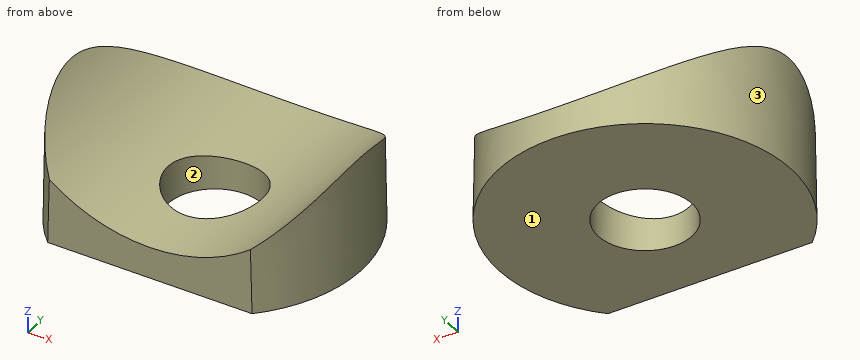
```python
from build123d import *

# Parameters (mm, degrees)
F0_R     = 14
F1_DEPTH = 12
F1_TAPER = 1
F2_R     = 16
F3_DEPTH = 16
F4_R     = 4.5
F5_DEPTH = 5
F7_DEPTH = 10.9201391502


with BuildPart() as f1:
    # F0 (on Top) → F1 (new body)
    with BuildSketch(Plane.XY):
        Circle(F0_R)
    extrude(amount=F1_DEPTH, taper=F1_TAPER)

    # F2 (on Front) → F3 (cut, symmetric)
    with BuildSketch(Plane.XZ):
        with Locations((0, 19)):
            Circle(F2_R)
    extrude(amount=F3_DEPTH, both=True, mode=Mode.SUBTRACT)

    # F4 (on face) → F5 (cut)
    with BuildSketch(Plane(origin=(0, 0, 0), x_dir=(1, 0, 0), z_dir=(0, 0, -1))):
        Circle(F4_R)
    extrude(amount=-F5_DEPTH, mode=Mode.SUBTRACT)

    # F6 (on face) → F7 (cut, through all)
    with BuildSketch(Plane(origin=(0, 0, 0), x_dir=(1, 0, 0), z_dir=(0, 0, -1))):
        with BuildLine():
            ThreePointArc((9.7979589711, 10), (0, 14), (-9.7979589711, 10))
            Line((-9.7979589711, 10), (9.7979589711, 10))
        make_face()
    extrude(amount=-F7_DEPTH, mode=Mode.SUBTRACT)


solid = f1.part
```
Here's how the part is built. I have some questions about the finished solid (model axes, mm). Face numbers are marked on the shaded views. Coordinates: 2 decimals unless noted, no trailing zeros. Order: outer loops, then holes, each group sorted by start corner. A loop starts at its lowest first (then second) coordinate and runs counter-clockwise, first axis right, second up.
1) Imagine slicing it at B-B on z = 7.5. List the corners of the cut face in (x, y) for me, and give its area (3 significant figures).
2) Imagine slicing it at A-A on z = 4.25. List the corners of the cut face in (x, y) for me, and give its area (3 significant figures).
3) We'd pull the mould along Y, two halves only. Please class the marked faces 1, 2 and 3: +Y half, -Y half, draft (parallel to the pull), parting line (faces both ways), or undercut.
4) Will these pins go through, and if not, where does the flat tip stop? pin 1 (2 mm diameter, centred on x = 11, y = 1, fed in from +Z); pin 2 (4 mm diameter, centred on x = 6.5, y = -7.5, fed in from +Z); pin 3 (2 mm diameter, centred on y = 5.5, z = 7.5, fed in from +X); pin 4 (3 mm diameter, centred on x = 8, z = 7, fed in from +Y).
5) I need wall thicknesses on line 1 (Y direction, x = 0, z = 2.75); line 2 (X direction, y = -1.5, z = 1.25). Which ranges of each line are inside material? Lowest first, please.
Response values:
1. outline: (-11.12, -8.28) - (-11.12, 8.28) arc R13.87 ccw to start; (11.12, -8.28) arc R13.87 ccw to (11.12, 8.28) - close
1. area: 61.9 mm2
2. outline: (-9.69, -10) - (-6.2, -10) - (-6.2, 12.47) arc R13.93 ccw to start; (6.2, -10) - (9.69, -10) arc R13.93 ccw to (6.2, 12.47) - close
2. area: 266 mm2
3. face 1: draft
3. face 2: undercut
3. face 3: parting line
4. pin 1: stops at z = 8.42
4. pin 2: stops at z = 5.44
4. pin 3: stops at x = 13.12
4. pin 4: passes through
5. line 1: y = -10 to -4.5, 4.5 to 13.95
5. line 2: x = -13.9 to -4.24, 4.24 to 13.9
